CAD build for the part. Positions are in the model's coordinates, mm. A direction names the side the tool comes from. Give positions to 0.01 mm unless a question says otherwise; leave off trailing zeros. Order: outer loops, then holes, each group sorted by start corner. A loop starts at its lowest first (then second) coordinate and runs counter-clockwise, first axis right, second up.
Item 1: Which spindle directions (+Z, -Z, +X, -X, +Y, -Y) get a long thin tool onto all of the face, cutting with end or side? Do faces 1 (the flat face through (-137.4, -137.4, 6.35)), 2 (the flat face through (-1, 1, 6.35)), 3 (the flat face through (-2, 120.65, 19)). Say none if no direction does.
Item 2: Band-saw the part on C-C on y = 40.5. Give the cut face in (x, z).
Item 3: Wall check: L1, parallel to Y at x = -133.35, z = 8; L2, parallel to Y at x = 0, z = 24.25. Give the ranges that are in metal, low to high.
Item 4: Two-plate mould, pull along X, no slides. Class faces 4 (the flat face through (-120.65, -2, 19)), 5 (the flat face through (-137.4, 129.3, 6.35)), 6 (the flat face through (152.4, -2, 6)), 7 (the flat face through (-109, 2, 25.4)): released by +X, released by -X, zero draft, split by the parting line, or undercut.
Item 5: Band-saw the part on A-A on x = 133.35. Give the cut face in (y, z).
Item 6: Flat gauge pins, fed straight in: P1, Ø4, axis at x = -24.5, z = 19.5, coming from the +Y side; P2, Ø3, axis at x = -0.5, y = -24, coming from the +Z side; P3, Ø4, axis at y = -14.5, z = 18.5, coming from the +X side. Where does each tip first touch, or does it go through?
```python
from build123d import *

# Parameters (mm, degrees)
F0_W     = 304.8
F0_H     = 304.8
F1_DEPTH = 25.4
F3_DEPTH = 19.05
F4_W     = 304.8
F4_H     = 304.8
F4_W_2   = 241.3
F4_H_2   = 241.3
F5_DEPTH = 12.7
F7_D     = 11.1125
F9_DEPTH = 6.35


with BuildPart() as f1:
    # F0 (on Top) → F1 (new body)
    with BuildSketch(Plane.XY):
        Rectangle(F0_W, F0_H)
    extrude(amount=F1_DEPTH)

    # F2 (on face) → F3 (cut)
    with BuildSketch(Plane.XY.offset(25.4)):
        with BuildLine():
            Line((98.8314, 105.1814), (-98.8314, 105.1814))
            ThreePointArc((-98.8314, 105.1814), (-103.321528, 103.321528), (-105.1814, 98.8314))
            Line((-105.1814, 98.8314), (-105.1814, -98.8314))
            ThreePointArc((-105.1814, -98.8314), (-103.321528, -103.321528), (-98.8314, -105.1814))
            Line((-98.8314, -105.1814), (98.8314, -105.1814))
            ThreePointArc((98.8314, -105.1814), (103.321528, -103.321528), (105.1814, -98.8314))
            Line((105.1814, -98.8314), (105.1814, 98.8314))
            ThreePointArc((105.1814, 98.8314), (103.321528, 103.321528), (98.8314, 105.1814))
        make_face()
    extrude(amount=-F3_DEPTH, mode=Mode.SUBTRACT)

    # F4 (on face) → F5 (cut)
    with BuildSketch(Plane.XY.offset(25.4)):
        Rectangle(F4_W, F4_H)
        Rectangle(F4_W_2, F4_H_2, mode=Mode.SUBTRACT)
    extrude(amount=-F5_DEPTH, mode=Mode.SUBTRACT)

    # F7 (through all)
    with Locations(Plane.XY.offset(12.7)):
        with Locations((-133.35, 133.35), (133.35, 133.35), (133.35, -133.35), (-133.35, -133.35)):
            Hole(F7_D / 2)

    # F8 (on face) → F9 (cut)
    with BuildSketch(Plane(origin=(0, 0, 0), x_dir=(1, 0, 0), z_dir=(0, 0, -1))):
        with BuildLine():
            Line((-140.49375, 124.61875), (-126.20625, 124.61875))
            ThreePointArc((-126.20625, 124.61875), (-125.083718, 125.083718), (-124.61875, 126.20625))
            Line((-124.61875, 126.20625), (-124.61875, 140.49375))
            ThreePointArc((-124.61875, 140.49375), (-125.083718, 141.616282), (-126.20625, 142.08125))
            Line((-126.20625, 142.08125), (-140.49375, 142.08125))
            ThreePointArc((-140.49375, 142.08125), (-141.616282, 141.616282), (-142.08125, 140.49375))
            Line((-142.08125, 140.49375), (-142.08125, 126.20625))
            ThreePointArc((-142.08125, 126.20625), (-141.616282, 125.083718), (-140.49375, 124.61875))
        make_face()
        with BuildLine():
            ThreePointArc((124.61875, 126.20625), (125.083718, 125.083718), (126.20625, 124.61875))
            Line((126.20625, 124.61875), (140.49375, 124.61875))
            ThreePointArc((140.49375, 124.61875), (141.616282, 125.083718), (142.08125, 126.20625))
            Line((142.08125, 126.20625), (142.08125, 140.49375))
            ThreePointArc((142.08125, 140.49375), (141.616282, 141.616282), (140.49375, 142.08125))
            Line((140.49375, 142.08125), (126.20625, 142.08125))
            ThreePointArc((126.20625, 142.08125), (125.083718, 141.616282), (124.61875, 140.49375))
            Line((124.61875, 140.49375), (124.61875, 126.20625))
        make_face()
        with BuildLine():
            ThreePointArc((124.61875, -140.49375), (125.083718, -141.616282), (126.20625, -142.08125))
            Line((126.20625, -142.08125), (140.49375, -142.08125))
            ThreePointArc((140.49375, -142.08125), (141.616282, -141.616282), (142.08125, -140.49375))
            Line((142.08125, -140.49375), (142.08125, -126.20625))
            ThreePointArc((142.08125, -126.20625), (141.616282, -125.083718), (140.49375, -124.61875))
            Line((140.49375, -124.61875), (126.20625, -124.61875))
            ThreePointArc((126.20625, -124.61875), (125.083718, -125.083718), (124.61875, -126.20625))
            Line((124.61875, -126.20625), (124.61875, -140.49375))
        make_face()
        with BuildLine():
            Line((-140.49375, -142.08125), (-126.20625, -142.08125))
            ThreePointArc((-126.20625, -142.08125), (-125.083718, -141.616282), (-124.61875, -140.49375))
            Line((-124.61875, -140.49375), (-124.61875, -126.20625))
            ThreePointArc((-124.61875, -126.20625), (-125.083718, -125.083718), (-126.20625, -124.61875))
            Line((-126.20625, -124.61875), (-140.49375, -124.61875))
            ThreePointArc((-140.49375, -124.61875), (-141.616282, -125.083718), (-142.08125, -126.20625))
            Line((-142.08125, -126.20625), (-142.08125, -140.49375))
            ThreePointArc((-142.08125, -140.49375), (-141.616282, -141.616282), (-140.49375, -142.08125))
        make_face()
    extrude(amount=-F9_DEPTH, mode=Mode.SUBTRACT)


solid = f1.part
```
The answers:
1. face 1: -Z
1. face 2: +Z
1. face 3: +Z, +X, -X, +Y
2. outline: (-152.4, 0) - (152.4, 0) - (152.4, 12.7) - (120.65, 12.7) - (120.65, 25.4) - (105.18, 25.4) - (105.18, 6.35) - (-105.18, 6.35) - (-105.18, 25.4) - (-120.65, 25.4) - (-120.65, 12.7) - (-152.4, 12.7) - close
3. L1: y = -152.4 to -138.91, -127.79 to 127.79, 138.91 to 152.4
3. L2: y = -120.65 to -105.18, 105.18 to 120.65
4. face 4: released by -X
4. face 5: undercut
4. face 6: released by +X
4. face 7: zero draft
5. outline: (-152.4, 0) - (-142.08, 0) - (-142.08, 6.35) - (-138.91, 6.35) - (-138.91, 12.7) - (-152.4, 12.7) - close; (-127.79, 6.35) - (-124.62, 6.35) - (-124.62, 0) - (124.62, 0) - (124.62, 6.35) - (127.79, 6.35) - (127.79, 12.7) - (-127.79, 12.7) - close; (138.91, 6.35) - (142.08, 6.35) - (142.08, 0) - (152.4, 0) - (152.4, 12.7) - (138.91, 12.7) - close
6. P1: stops at y = 120.65
6. P2: stops at z = 6.35
6. P3: stops at x = 120.65
